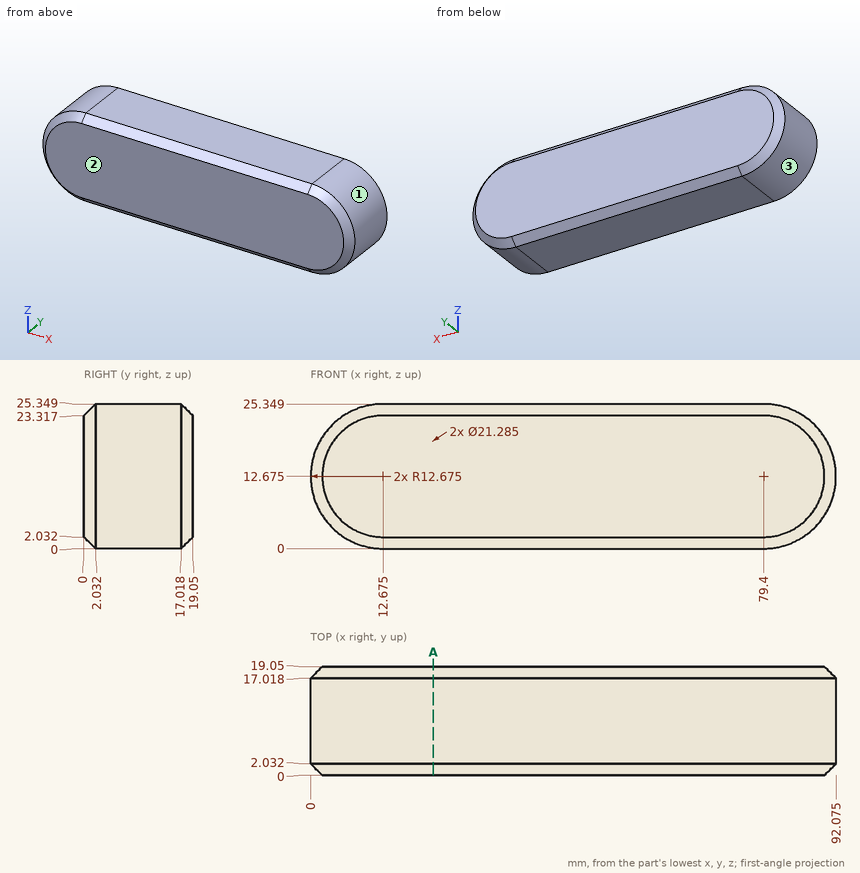
For this review, use the dimensioned drawing (mm, ordinates from the lowest corner) and the shaded views. Round coordinates to 2 decimals unless told otherwise and drop trailing zeros. Write each loop counter-clockwise with the first axis right and the second up, starting at its lowest first coordinate (ties: lowest second). Pieces come first, ordered by that corner, then holes. Notation, with made-up numbers: (-30, -10.5) - (8, -10.5) arc R25 ccw to (8, 19.5) - close; hole circle Ø7 at (-10, 34.5). An arc over 180 degrees is marked (long way). Answer as a JSON object with one key per item and string values.
1. We need section A-A on x = 21.5. Give the boundary of the cut face in (y, z), then the cut area to 3 significant figures.
Response values:
{"outline": "(0, 2.03) - (2.03, 0) - (17.02, 0) - (19.05, 2.03) - (19.05, 23.32) - (17.02, 25.35) - (2.03, 25.35) - (0, 23.32) - close", "area": "475 mm2"}
2. To check wall thickness, follow line 1 along X through (y, z) = (11, 12); line 2 along Z through (x, y) = (80, 6.5) (1 decimal); line 3 along X through (y, z) = (14, 10.5). State the ranges of each line that lie inside material, in increasing order.
Response values:
{"line 1": "x = 0.02 to 92.06", "line 2": "z = 0 to 25.3", "line 3": "x = 0.19 to 91.89"}
3. For pin 1 Ø8 at (y, z) = (5, 17.5) entering from +X; pin 2 Ø3 at (y, z) = (4, 4.5) entering from +X (1 decimal), all flat-tipped, find the tip position at first contact; note any pin that passes through.
Response values:
{"pin 1": "stops at x = 92.05", "pin 2": "stops at x = 90.2"}
4. Draft analysis for pull direction X (two halves, no side actions). For the marked faces 1, 2 and 3, state which applies: +X half, -X half, draft (parallel to the pull), parting line (faces both ways), or undercut.
Response values:
{"face 1": "+X half", "face 2": "draft", "face 3": "-X half"}
